from build123d import *


with BuildPart() as f1:
    # F0 (on Front) → F1 (revolve)
    with BuildSketch(Plane.XZ):
        with BuildLine():
            Line((0, 8), (0, 0))
            Line((0, 0), (124.24945, 0))
            ThreePointArc((124.24945, 0), (140.63249, 8.528471), (143.043302, 26.840403))
            Line((143.043302, 26.840403), (60, 255))
            Line((60, 255), (60, 300))
            Line((60, 300), (52, 300))
            Line((52, 300), (52, 253.589384))
            Line((52, 253.589384), (135.525761, 24.104242))
            ThreePointArc((135.525761, 24.104242), (134.079274, 13.117083), (124.24945, 8))
            Line((124.24945, 8), (0, 8))
        make_face()
    revolve(axis=Axis((0, 0, 4), (0, 0, 1)))


solid = f1.part
Input: part model. Units: mm. Frame: model coordinates. A direction names the side the tool comes from. Coordinates: 2 decimals unless noted, no trailing zeros. Loops run counter-clockwise (first coordinate to the right, second up) from the corner with the lowest first, then second, coordinate; pieces in that order, holes last. Notation, with made-up numbers: (62.25, 4.25) -> (97.25, 4.25) arc R25 cw to (97.25, 30.25) -> close; hole circle Ø4 at (10.25, 18.5). An arc over 180 degrees is marked (long way). Write item = value, one per line. Start each with the question number.
Item 1: Mould query, pull axis Y, two halves, no side actions, for faces 1 (the face through (-18, 49, 300)), 2 (the face through (-41.265, -31.641, 276.47)), 3 (the face through (-19.88, -89.53, 167.87)). Classes: pulls with the +Y half, pulls with the -Y half, needs draft (parallel to the pull), parting line crosses it, or undercut.
Item 2: Reachability of faces 4 (the face through (-59.94, 2.64, 277.82)), 5 (the face through (2, 2, 0)), 6 (the face through (-18.441, -83.044, 162.739)) from +Z, -Z, +X, -X, +Y, -Y: full face, straight path, thin tool, end or side. Return the list, or none.
Item 3: Material intervals for line 1 (Y direction, x = 0, z = 265); line 2 (Z direction, x = 33, y = 43.5); line 3 (Z direction, x = -4, y = 45.5), sorted ascending.
Item 4: First-contact query: P1, Ø1.5, axis at y = -10.5, z = 147.5, coming from the -X side; P2, Ø12, axis at x = -106.5, z = 66.5, coming from the +Y side; P3, Ø4, axis at x = 81, z = 62.5, coming from the +Y side. Flat tips, straight axial feed; report the tip coordinate or a pass-through.
Item 5: Cut plane A-A, the plane y = 0. Return loops of the section in (x, z).
Item 6: Cut plane C-C, the plane z = 38.5. Return loops of the section in (x, y).
Item 7: Cut plane D-D, the plane z = 236. Return loops of the section in (x, y).
Ans:
q1.face_1 = needs draft
q1.face_2 = undercut
q1.face_3 = parting line crosses it
q2.face_4 = +Z
q2.face_5 = -Z, +X, -X, +Y, -Y
q2.face_6 = none
q3.line_1 = -60 to -52, 52 to 60
q3.line_2 = 0 to 8, 246.44 to 300
q3.line_3 = 0 to 8
q4.P1 = -98.85
q4.P2 = 81.02
q4.P3 = 103.58
q5.outline = (-143.04, 26.84) arc R20 ccw to (-124.25, 0) -> (124.25, 0) arc R20 ccw to (143.04, 26.84) -> (60, 255) -> (60, 300) -> (52, 300) -> (52, 253.59) -> (135.53, 24.1) arc R12 cw to (124.25, 8) -> (-124.25, 8) arc R12 cw to (-135.53, 24.1) -> (-52, 253.59) -> (-52, 300) -> (-60, 300) -> (-60, 255) -> close
q6.outline = circle Ø277.6 at (0, 0); hole circle Ø260.57 at (0, 0)
q7.outline = circle Ø133.83 at (0, 0); hole circle Ø116.8 at (0, 0)
